```python
from build123d import *

# Parameters (mm, degrees)
SKETCH1_R           = 4.7625
BOSS_EXTRUDE1_DEPTH = 16
SKETCH2_R           = 21
BOSS_EXTRUDE2_DEPTH = 5.588
BOSS_EXTRUDE3_DEPTH = 2.54
SKETCH6_R           = 1.55
CUT_EXTRUDE1_DEPTH  = 19.54
SKETCH7_R           = 1.45
CUT_EXTRUDE2_DEPTH  = 7.62
SKETCH8_R           = 6
SKETCH8_R_2         = 4
BOSS_EXTRUDE4_DEPTH = 11
FILLET1_R           = 2


with BuildPart() as part:
    # Sketch1 → Boss-Extrude1 (new body)
    with BuildSketch(Plane.XY):
        Circle(SKETCH1_R)
    extrude(amount=-BOSS_EXTRUDE1_DEPTH)

    # Sketch2 → Boss-Extrude2 (add)
    with BuildSketch(Plane.XY):
        Circle(SKETCH2_R)
    extrude(amount=-BOSS_EXTRUDE2_DEPTH)

    # Sketch3 → Boss-Extrude3 (add)
    with BuildSketch(Plane(origin=(0, 0, -16), x_dir=(-1, 0, 0), z_dir=(0, 0, -1))):
        with BuildLine():
            Line((1.979898987, -1.979898987), (3.367596045, -3.367596045))
            ThreePointArc((3.367596045, -3.367596045), (4.399976274, -1.822529847), (4.7625, 0))
            Line((4.7625, 0), (2.8, 0))
            ThreePointArc((2.8, 0), (2.586862691, -1.071513611), (1.979898987, -1.979898987))
        make_face()
        with BuildLine():
            ThreePointArc((-3.367596045, 3.367596045), (-4.399976274, 1.822529847), (-4.7625, 0))
            Line((-4.7625, 0), (-2.8, 0))
            ThreePointArc((-2.8, 0), (-2.586862691, 1.071513611), (-1.979898987, 1.979898987))
            Line((-1.979898987, 1.979898987), (-3.367596045, 3.367596045))
        make_face()
        with BuildLine():
            ThreePointArc((-3.367596045, -3.367596045), (-1.822529847, -4.399976274), (0, -4.7625))
            Line((0, -4.7625), (0, -2.8))
            ThreePointArc((0, -2.8), (-1.071513611, -2.586862691), (-1.979898987, -1.979898987))
            Line((-1.979898987, -1.979898987), (-3.367596045, -3.367596045))
        make_face()
        with BuildLine():
            Line((0, 4.7625), (0, 2.8))
            ThreePointArc((0, 2.8), (1.071513611, 2.586862691), (1.979898987, 1.979898987))
            Line((1.979898987, 1.979898987), (3.367596045, 3.367596045))
            ThreePointArc((3.367596045, 3.367596045), (1.822529847, 4.399976274), (0, 4.7625))
        make_face()
    extrude(amount=BOSS_EXTRUDE3_DEPTH)

    # Sketch6 → Cut-Extrude1 (cut, through all)
    with BuildSketch(Plane.XY):
        Circle(SKETCH6_R)
    extrude(amount=-CUT_EXTRUDE1_DEPTH, mode=Mode.SUBTRACT)

    # Sketch7 → Cut-Extrude2 (cut)
    with BuildSketch(Plane.XY):
        with Locations((-16, 0)):
            Circle(SKETCH7_R)
    extrude(amount=-CUT_EXTRUDE2_DEPTH, mode=Mode.SUBTRACT)

    # Sketch8 → Boss-Extrude4 (add)
    with BuildSketch(Plane.XY):
        Circle(SKETCH8_R)
        Circle(SKETCH8_R_2, mode=Mode.SUBTRACT)
    extrude(amount=BOSS_EXTRUDE4_DEPTH)

    # Fillet1
    fillet1_edges = [part.edges().sort_by_distance(p)[0] for p in [
        (-4.7625, 0, -5.588),
    ]]
    fillet(fillet1_edges, radius=FILLET1_R)


solid = part.part
```
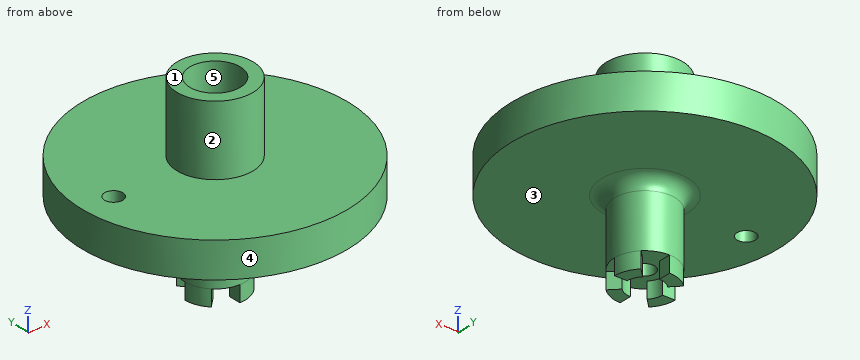
Here's how the part is built. I have some questions about the finished solid (model axes, mm). Face numbers are marked on the shaded views. A direction names the side the tool comes from. Coordinates: 2 decimals unless noted, no trailing zeros. Loops run counter-clockwise (first coordinate to the right, second up) from the corner with the lowest first, then second, coordinate; pieces in that order, holes last. Notation, with made-up numbers: (-27, -4.5) - (19, -4.5) arc R19 cw to (19, 3.5) - close; hole circle Ø10 at (-24, -18.5). An arc over 180 degrees is marked (long way). Return JSON: item names as keys, results as strings. Group by question number.
Item 1: On a 3-axis mill with a long thin cutter (end or side, diameter ignored), from which of +Z, -Z, +X, -X, +Y, -Y can I reach the whole of each face in a straight line? I mean the marked faces 1 and 2. Say none if no direction works.
Item 2: I need wall thicknesses on line 1 (Y direction, x = 0, z = -10.5); line 2 (Y direction, x = 0, z = 8.5); line 3 (Z direction, x = -4, y = -13). Which ranges of each line are inside material? Lowest first, please. Write a range as from..to.
Item 3: Will these pins go through, and if not, where does the flat tip stop? P1, Ø3, axis at x = 0, y = 0, coming from the -Z side; P2, Ø1.6, axis at y = 4, z = -18, coming from the +X side; P3, Ø6.5, axis at x = 0, y = 0, coming from the -Z side; P4, Ø1, axis at x = -12, y = 11, coming from the +Z side.
Item 4: If we section it at D-D on y = -9: Write out the boundary of the cut face in (x, z), and give its area (3 significant figures).
Item 5: We'd pull the mould along X, two halves only. Please class the marked faces 3, 4 and 5: +X half, -X half, draft (parallel to the pull), parting line (faces both ways), or undercut.
Item 6: If we section it at C-C on z = -1.5: Write out the boundary of the cut face in (x, y), and give its area (3 significant figures).
Item 7: If we section it at A-A on x = -16: Write out the boundary of the cut face in (y, z), and give its area (3 significant figures).
Item 8: If we section it at B-B on z = 6: Write out the boundary of the cut face in (x, y), and give its area (3 significant figures).
Calculated:
{
 "1": {"face 1": "+Z, +X, -X, +Y, -Y", "face 2": "+Z"},
 "2": {"line 1": "y = -4.76..-1.55, 1.55..4.76", "line 2": "y = -6..-4, 4..6", "line 3": "z = -5.59..0"},
 "3": {"P1": "passes through", "P2": "stops at x = 3.53", "P3": "stops at z = -18.54", "P4": "stops at z = 0"},
 "4": {"outline": "(-18.97, -5.59) - (18.97, -5.59) - (18.97, 0) - (-18.97, 0) - close", "area": "212 mm^2"},
 "5": {"face 3": "draft", "face 4": "parting line", "face 5": "undercut"},
 "6": {"outline": "circle Ø42 at (0, 0); hole circle Ø2.9 at (-16, 0); hole circle Ø3.1 at (0, 0)", "area": "1,370 mm^2"},
 "7": {"outline": "(-13.6, -5.59) - (-1.45, -5.59) - (-1.45, 0) - (-13.6, 0) - close; (1.45, -5.59) - (13.6, -5.59) - (13.6, 0) - (1.45, 0) - close", "area": "136 mm^2"},
 "8": {"outline": "circle Ø12 at (0, 0); hole circle Ø8 at (0, 0)", "area": "62.8 mm^2"}
}
